The listing builds one solid part. Answer for the finished solid, in the listing's coordinates (mm). Face numbers are marked on the shaded views. A direction names the side the tool comes from. Coordinates: 2 decimals unless noted, no trailing zeros. Loops run counter-clockwise (first coordinate to the right, second up) from the corner with the lowest first, then second, coordinate; pieces in that order, holes last. Notation, with made-up numbers: (-21.5, 84) - (-0.5, 84) arc R31 ccw to (-0.5, 118) - close; hole circle Ø5 at (-9, 34.5). An arc over 180 degrees is marked (long way). Write each question's results on one line, items separated by ' | '. Start each with the question number.
(1) Determine the mould class of the marked faces 3, 4 and 5 for opening direction Y: released by +Y, released by -Y, zero draft, split by the parting line, or undercut.
(2) Given pin 1 Ø8 at (x, z) = (5, 34.5) entering from -Y; pin 2 Ø2 at (y, z) = (38.5, 48.5) entering from +X; pin 3 Ø1 at (x, y) = (31, 28.5) entering from +Z; pin 4 Ø3 at (y, z) = (-50.5, 39.5) entering from -X, each flat-ended and moving along its own axis, determine where each tip first touches the part or whether it passes through.
(3) Consider line 1 (Y direction, x = 0, z = 12.5); line 2 (Y direction, x = -3, z = 35); line 3 (X direction, y = -53.5, z = 23.5). Determine where each line is inside the solid, lowest interval first. Write a range as from..to.
(4) Find section A-A on x = 0. Determine the outline of the cut face in (y, z), then the cut area to 3 significant figures.
(5) Find section C-C on z = -3. Determine the outline of the cut face in (x, y).
(6) Find section B-B on y = 4.5. Determine the outline of the cut face in (x, z), then the cut area to 3 significant figures.
(7) For the marked faces 1 and 2, determine the directions among +Z, -Z, +X, -X, +Y, -Y from which every point of the face is accessible in a straight line to the end or side of a thin tool.
from build123d import *

# Parameters (mm, degrees)
SKETCH1_R           = 40
SKETCH1_R_2         = 35
BOSS_EXTRUDE1_DEPTH = 50
BOSS_EXTRUDE2_START = -50
BOSS_EXTRUDE2_DEPTH = 50
SCALE1_SCALE        = 1.5


with BuildPart() as part:
    # Sketch1 → Boss-Extrude1 (new body)
    with BuildSketch(Plane.XY):
        Circle(SKETCH1_R)
        Circle(SKETCH1_R_2, mode=Mode.SUBTRACT)
    extrude(amount=BOSS_EXTRUDE1_DEPTH)

    # Sketch2 → Boss-Extrude2 (add)
    with BuildSketch(Plane.XY.offset(50).offset(BOSS_EXTRUDE2_START)):
        with BuildLine():
            Line((0, 40), (0, 50.63587493))
            Line((0, 50.63587493), (-40, 50.63587493))
            ThreePointArc((-40, 50.63587493), (-38.47413578, 35.580764102), (-33.958601629, 21.137960531))
            ThreePointArc((-33.958601629, 21.137960531), (-19.422687491, 34.967974071), (0, 40))
        make_face()
        with BuildLine():
            ThreePointArc((33.958601629, 21.137960531), (38.47413578, 35.580764102), (40, 50.63587493))
            Line((40, 50.63587493), (0, 50.63587493))
            Line((0, 50.63587493), (0, 40))
            ThreePointArc((0, 40), (19.422687491, 34.967974071), (33.958601629, 21.137960531))
        make_face()
    extrude(amount=BOSS_EXTRUDE2_DEPTH)


with BuildPart() as part_1:
    # Scale1: scaled about (0, 21.957707066, 25)
    add(part.part.scale(SCALE1_SCALE).moved(Location((0, -10.978853533, -12.5))))


solid = part_1.part
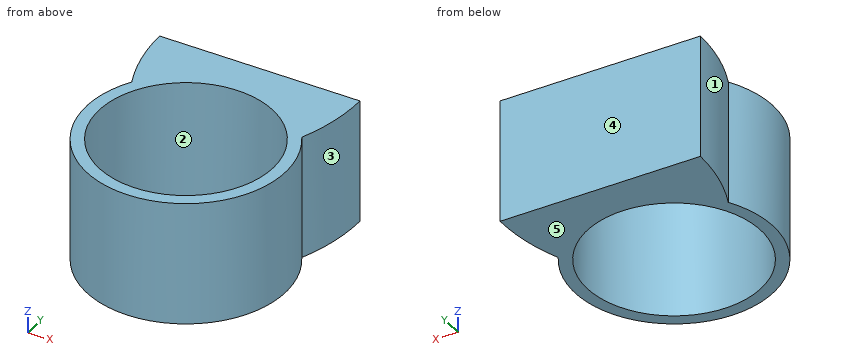
Values:
1) face 3: undercut | face 4: released by +Y | face 5: zero draft
2) pin 1: stops at y = -70.97 | pin 2: stops at x = 57.08 | pin 3: passes through | pin 4: stops at x = -46.42
3) line 1: y = -70.98..-63.48, 41.52..64.97 | line 2: y = -70.9..-63.39, 41.44..64.97 | line 3: x = -42.33..-30.79, 30.79..42.33
4) outline: (-70.98, -12.5) - (-63.48, -12.5) - (-63.48, 62.5) - (-70.98, 62.5) - close; (41.52, -12.5) - (64.97, -12.5) - (64.97, 62.5) - (41.52, 62.5) - close | area: 2,320 mm²
5) outline: (-60, 64.97) arc R112.55 ccw to (-50.94, 20.73) arc R60 ccw (long way) to (50.94, 20.73) arc R112.55 ccw to (60, 64.97) - close; hole circle Ø105 at (0, -10.98)
6) outline: (-57.97, -12.5) - (-50.17, -12.5) - (-50.17, 62.5) - (-57.97, 62.5) - close; (50.17, -12.5) - (57.97, -12.5) - (57.97, 62.5) - (50.17, 62.5) - close | area: 1,170 mm²
7) face 1: +Z, -Z, -X | face 2: +Z, -Z
